from build123d import *

# Parameters (mm, degrees)
SKETCH2_W           = 30
SKETCH2_H           = 30
BOSS_EXTRUDE1_DEPTH = 50
SKETCH3_W           = 25
SKETCH3_H           = 25
CUT_EXTRUDE1_DEPTH  = 2.5
FILLET1_R           = 5
CIRPATTERN1_COUNT   = 4


with BuildPart() as part:
    # Sketch2 → Boss-Extrude1 (new body)
    with BuildSketch(Plane(origin=(0, 0, 0), x_dir=(1, 0, 0), z_dir=(0, 1, 0))):
        Rectangle(SKETCH2_W, SKETCH2_H)
    extrude(amount=BOSS_EXTRUDE1_DEPTH)

    # Sketch3 → Cut-Extrude1 (cut)
    with BuildSketch(Plane(origin=(0, 50, 0), x_dir=(1, 0, 0), z_dir=(0, 1, 0))):
        Rectangle(SKETCH3_W, SKETCH3_H)
    extrude(amount=-CUT_EXTRUDE1_DEPTH, mode=Mode.SUBTRACT)

    # Fillet1
    fillet1_edges = [part.edges().sort_by_distance(p)[0] for p in [
        (15, 25, 15),
        (-15, 25, 15),
        (-15, 25, -15),
        (15, 25, -15),
    ]]
    fillet(fillet1_edges, radius=FILLET1_R)

    # Cut-Loft2: read off the stored shape, not the designer's step
    # Cut-Loft2: loft between two sections, ruled curve by curve
    cut_loft2_from = [
        Edge.make_bspline([(0, 0, -12.5), (-25, 0, -12.5), (-25, 0, 12.5), (0, 0, 12.5), (25, 0, 12.5), (25, 0, -12.5), (0, 0, -12.5)], [0, 0, 0, 0, 0.5, 0.5, 0.5, 1, 1, 1, 1], 3, [1, 0.333333333, 0.333333333, 1, 0.333333333, 0.333333333, 1]),
    ]
    cut_loft2_to = [
        Edge.make_bspline([(0.784484005, 47.5, -2.373728048), (-3.962972092, 47.5, -3.942696057), (-5.531940101, 47.5, 0.804760039), (-0.784484005, 47.5, 2.373728048), (3.962972092, 47.5, 3.942696057), (5.531940101, 47.5, -0.804760039), (0.784484005, 47.5, -2.373728048)], [0, 0, 0, 0, 0.5, 0.5, 0.5, 1, 1, 1, 1], 3, [1, 0.333333333, 0.333333333, 1, 0.333333333, 0.333333333, 1]),
    ]
    cut_loft2 = Solid(Shell([*[Face.make_surface_from_curves(cut_loft2_from[k], cut_loft2_to[k]) for k in range(1)], Face(Wire(cut_loft2_from)), Face(Wire(cut_loft2_to))]))
    add(cut_loft2, mode=Mode.SUBTRACT)

    # Cut-Sweep1: sweep along a curve in space
    with BuildLine() as cut_sweep1_path:
        Line((-10, 50, 15), (10, 50, 15))
    # Sketch9 → Cut-Sweep1 (sweep, cut)
    with BuildSketch(Plane.ZY):
        Polygon((15, 41), (12, 33), (15, 25), align=None)
    cut_sweep1 = sweep(path=cut_sweep1_path.line, mode=Mode.SUBTRACT)

    # CirPattern1: Cut-Sweep1 ×4 about axis
    cirpattern1_axis = Axis((0, 0, 0), (0, 1, 0))
    for i in range(1, CIRPATTERN1_COUNT):
        add(cut_sweep1.rotate(cirpattern1_axis, i * 360 / CIRPATTERN1_COUNT), mode=Mode.SUBTRACT)


solid = part.part
CAD build for the part. Positions are in the model's coordinates, mm. A direction names the side the tool comes from. Coordinates: 2 decimals unless noted, no trailing zeros. Answer as a JSON object with one key per item and string values. Group by question number.
1) Pin check, flat tips, straight feed: pin 1 Ø3.5 at (y, z) = (34, 13.5) entering from +X; pin 2 Ø2.5 at (y, z) = (31.5, -13) entering from -X; pin 3 Ø1.5 at (y, z) = (36, 13.5) entering from -X. Stop position of each tip, or through.
2) Wall check: line 1 (Y direction, x = -10, z = -12); line 2 (X direction, y = 10, z = 7); line 3 (X direction, y = 44.5, z = 0). Give the ranges that are in metal, low to high. Write a range as from..to.
3) Tool access for faces 1 (the face through (-10, 33, 14)), 2 (the face through (0, 49, 12.5)), 3 (the face through (-10, 33, -14)), 4 (the face through (13.521, 37.056, -0.14)): list every direction of +Z, -Z, +X, -X, +Y, -Y with a clear straight run to the whole face (end or side of a thin tool).
4) Mould opens along Z. For faces 5 (the face through (15, 12, 0)), 6 (the face through (13, 25, 14)), 7 (the face through (14, 33, 10)), 8 (the face through (0, 47.5, -3)) say: +Z half, -Z half, draft (parallel to the pull), parting line (faces both ways), or undercut.
Values follow:
{
 "1": {"pin 1": "stops at x = 14.68", "pin 2": "stops at x = -14.68", "pin 3": "stops at x = -14.18"},
 "2": {"line 1": "y = 0..47.5", "line 2": "x = -15..-7.65, 7.65..15", "line 3": "x = -15..-3.1, 3.1..15"},
 "3": {"face 1": "+Z", "face 2": "+Y", "face 3": "-Z", "face 4": "+X"},
 "4": {"face 5": "draft", "face 6": "+Z half", "face 7": "undercut", "face 8": "undercut"}
}
